from build123d import *

# Parameters (mm, degrees)
F2_R     = 1
F3_R     = 0.75
F4_DEPTH = 4.5
F5_R     = 9.2
F5_R_2   = 8
F6_DEPTH = 4


with BuildPart() as f1:
    # F0 (on Front) → F1 (revolve)
    with BuildSketch(Plane.XZ):
        Polygon((0, 16.2), (0, 0), (8, 0), (8, 8.8), (9.2, 8.8), (9.2, 10.6), (8, 10.6), (8, 16.2), align=None)
    revolve(axis=Axis((0, 0, 8.1), (0, 0, 1)))

    # F2
    f2_edges = [f1.edges().sort_by_distance(p)[0] for p in [
        (-8, 0, 0),
    ]]
    fillet(f2_edges, radius=F2_R)

    # F3 (on face) → F4 (join)
    with BuildSketch(Plane(origin=(0, 0, 0), x_dir=(1, 0, 0), z_dir=(0, 0, -1))):
        Circle(F3_R)
        with Locations((0, 5)):
            Circle(F3_R)
        with Locations((-3.909157, 3.117449)):
            Circle(F3_R)
        with Locations((-4.87464, -1.112605)):
            Circle(F3_R)
        with Locations((-2.169419, -4.504844)):
            Circle(F3_R)
        with Locations((2.169419, -4.504844)):
            Circle(F3_R)
        with Locations((4.87464, -1.112605)):
            Circle(F3_R)
        with Locations((3.909157, 3.117449)):
            Circle(F3_R)
    extrude(amount=F4_DEPTH)

    # F5 (on face) → F6 (join)
    with BuildSketch(Plane(origin=(0, 0, 8.8), x_dir=(1, 0, 0), z_dir=(0, 0, -1))):
        Polygon((9.5, -5.484828), (9.5, 5.484828), (0, 10.969655), (-9.5, 5.484828), (-9.5, -5.484828), (0, -10.969655), align=None)
        Circle(F5_R, mode=Mode.SUBTRACT)
        Circle(F5_R)
        Circle(F5_R_2, mode=Mode.SUBTRACT)
    extrude(amount=F6_DEPTH)


solid = f1.part
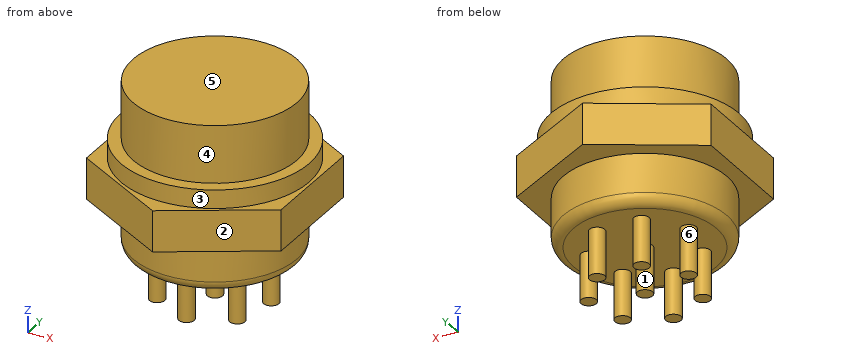
Design review of the part built by this model. Coordinates are the model's own, in mm. Face numbers are marked on the shaded views. A direction names the side the tool comes from. Round coordinates to 2 decimals unless told otherwise and drop trailing zeros. Write each loop counter-clockwise with the first axis right and the second up, starting at its lowest first coordinate (ties: lowest second). Pieces come first, ordered by that corner, then holes. Notation, with made-up numbers: (-28, 30.5) -> (-24, 30.5) arc R20 cw to (-24, 36.5) -> close; hole circle Ø9 at (-27, 72.25). An arc over 180 degrees is marked (long way). One line per item, written item: value. Start each with the question number.
Q1. To check wall thickness, follow probe 1 along X at (y, z) = (4.5, -3.5); probe 2 along Y at (x, z) = (-6.5, 11.75); probe 3 along Z at (x, y) = (4.5, 2.75). State the ranges of each line that lie inside material, in increasing order.
Q2. Add section D-D (z = 14). Give the boundary of the cut face in (x, y), then the cut area to 3 significant figures.
Q3. Insertion check: P1, Ø1.5, axis at x = -0.5, y = -3.5, coming from the -Z side; P2, Ø5, axis at x = -3, z = 1, coming from the +Y side; P3, Ø1, axis at x = 3, y = -8, coming from the -Z side. Each pin has a flat end and moves straight along its axis. Give the tip position at first contact, or say it passes through.
Q4. Add section A-A (y = 0). Give the boundary of the cut face in (x, z).
Q5. The part is to be moulded in two halves that separate along X. For the marked faces 4, 5 and 6, say which applies: pulls with the +X half, pulls with the -X half, needs draft (parallel to the pull), parting line crosses it, or undercut.
Q6. Tool access review of the marked faces 1, 2 and 3: name each direction out of +Z, -Z, +X, -X, +Y, -Y from which nothing blocks a thin tool from reaching the whole face with its end or side.
Q7. Add section C-C (z = -2.25). Give the boundary of the cut face in (x, y).
Q8. Add section B-B (z = 5.5). Give the boundary of the cut face in (x, y), then the cut area to 3 significant figures.
Response:
1. probe 1: x = -2.92 to -1.42, 1.42 to 2.92
1. probe 2: y = -4.66 to 4.66
1. probe 3: z = 0 to 16.2
2. outline: circle Ø16 at (0, 0)
2. area: 201 mm^2
3. P1: stops at z = 0
3. P2: stops at y = 7.98
3. P3: stops at z = 4.8
4. outline: (-9.5, 4.8) -> (-8, 4.8) -> (-8, 1) arc R1 ccw to (-7, 0) -> (-0.75, 0) -> (-0.75, -4.5) -> (0.75, -4.5) -> (0.75, 0) -> (7, 0) arc R1 ccw to (8, 1) -> (8, 4.8) -> (9.5, 4.8) -> (9.5, 8.8) -> (9.2, 8.8) -> (9.2, 10.6) -> (8, 10.6) -> (8, 16.2) -> (-8, 16.2) -> (-8, 10.6) -> (-9.2, 10.6) -> (-9.2, 8.8) -> (-9.5, 8.8) -> close
5. face 4: parting line crosses it
5. face 5: needs draft
5. face 6: undercut
6. face 1: -Z
6. face 2: +Z, -Z, +X, -Y
6. face 3: +Z
7. outline: circle Ø1.5 at (-4.87, 1.11); circle Ø1.5 at (-3.91, -3.12); circle Ø1.5 at (-2.17, 4.5); circle Ø1.5 at (0, -5); circle Ø1.5 at (0, 0); circle Ø1.5 at (2.17, 4.5); circle Ø1.5 at (3.91, -3.12); circle Ø1.5 at (4.87, 1.11)
8. outline: (-9.5, -5.48) -> (0, -10.97) -> (9.5, -5.48) -> (9.5, 5.48) -> (0, 10.97) -> (-9.5, 5.48) -> close
8. area: 313 mm^2
